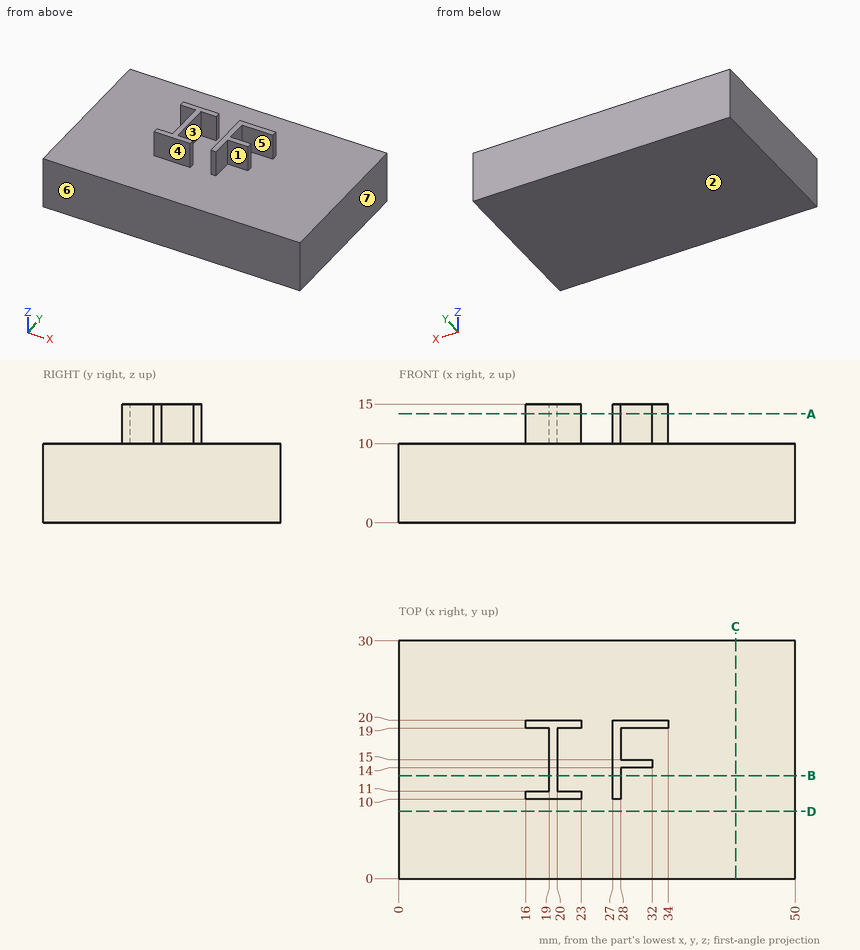
For this review, use the dimensioned drawing (mm, ordinates from the lowest corner) and the shaded views. A direction names the side the tool comes from. Round coordinates to 2 decimals unless told otherwise and drop trailing zeros. Loops run counter-clockwise (first coordinate to the right, second up) from the corner with the lowest first, then second, coordinate; pieces in that order, holes last. Notation, with made-up numbers: M 76,-2.75 L 111,-2.75 A8 cw 111,10.25 Z; hole C -15.75,82 d11. An arc over 180 degrees is marked long. Answer as CSV lines item,"result".
1. For the marked faces 1, 2, 3 and 4, list the 3-axis set-ups (+Z, -Z, +X, -X, +Y, -Y) from which the entire face can be reached by the end or side of a thin tool; tool diameter is ignored.
Outcome:
face 1,"+Z, +X, -Y"
face 2,"-Z, +X, -X, +Y, -Y"
face 3,"+Z"
face 4,"+Z, +X, -X, -Y"
2. We need section A-A (z = 13.75). Give the boundary of the cut face in (x, y), plus the area to 3 significant figures.
Outcome:
outline,"M 16,10 L 23,10 L 23,11 L 20,11 L 20,19 L 23,19 L 23,20 L 16,20 L 16,19 L 19,19 L 19,11 L 16,11 Z; M 27,10 L 28,10 L 28,14 L 32,14 L 32,15 L 28,15 L 28,19 L 34,19 L 34,20 L 27,20 Z"
area,"42.0 mm2"
3. Insertion check: pin 1 Ø1.1 at (y, z) = (10.5, 11.5) entering from +X; pin 2 Ø2.5 at (x, z) = (17.5, 11.5) entering from +Y; pin 3 Ø2.5 at (x, z) = (21.5, 13.5) entering from -Y. Each pin has a flat end and moves straight along its axis. Give the tip position at first contact, or say it passes through.
Outcome:
pin 1,"stops at x = 28"
pin 2,"stops at y = 20"
pin 3,"stops at y = 10"
4. We need section D-D (y = 8.5). Give the boundary of the cut face in (x, z).
Outcome:
outline,"M 0,0 L 50,0 L 50,10 L 0,10 Z"
5. We need section B-B (y = 13). Give the boundary of the cut face in (x, z).
Outcome:
outline,"M 0,0 L 50,0 L 50,10 L 28,10 L 28,15 L 27,15 L 27,10 L 20,10 L 20,15 L 19,15 L 19,10 L 0,10 Z"
6. We need section C-C (x = 42.5). Give the boundary of the cut face in (y, z).
Outcome:
outline,"M 0,0 L 30,0 L 30,10 L 0,10 Z"
7. Draft analysis for pull direction Y (two halves, no side actions). For the marked faces 5, 6 and 7, state which applies: pulls with the +Y half, pulls with the -Y half, needs draft (parallel to the pull), parting line crosses it, or undercut.
Outcome:
face 5,"undercut"
face 6,"pulls with the -Y half"
face 7,"needs draft"
8. To check wall thickness, follow L1, parallel to X at y = 13.75, z = 14.25; L2, parallel to X at y = 14.5, z = 12.25; L3, parallel to Y at x = 21.5, z = 11.25. State the ranges of each line that lie inside material, in increasing order. Write a range as [from, to].
Outcome:
L1,"x = [19, 20], [27, 28]"
L2,"x = [19, 20], [27, 32]"
L3,"y = [10, 11], [19, 20]"
